from build123d import *

# Parameters (mm, degrees)
F0_W     = 406.4
F0_H     = 431.8
F1_DEPTH = 431.8
F2_W     = 304.8
F2_H     = 330.2
F3_DEPTH = 1270
F4_W     = 304.8
F4_H     = 330.2
F5_DEPTH = 754.38
F6_W     = 330.2
F6_H     = 330.2
F7_DEPTH = 1270


with BuildPart() as f1:
    # F0 (on Top) → F1 (new body)
    with BuildSketch(Plane.XY):
        with Locations((142.597137, -170.802241)):
            Rectangle(F0_W, F0_H)
    extrude(amount=F1_DEPTH)

    # F2 (on face) → F3 (cut)
    with BuildSketch(Plane.XZ.offset(386.702241)):
        with Locations((142.597137, 215.9)):
            Rectangle(F2_W, F2_H)
    extrude(amount=-F3_DEPTH, mode=Mode.SUBTRACT)

    # F4 (on face) → F5 (cut)
    with BuildSketch(Plane(origin=(0, 0, 0), x_dir=(1, 0, 0), z_dir=(0, 0, -1))):
        with Locations((142.597137, 170.802241)):
            Rectangle(F4_W, F4_H)
    extrude(amount=-F5_DEPTH, mode=Mode.SUBTRACT)

    # F6 (on face) → F7 (cut)
    with BuildSketch(Plane.YZ.offset(345.797137)):
        with Locations((-170.802241, 215.9)):
            Rectangle(F6_W, F6_H)
    extrude(amount=-F7_DEPTH, mode=Mode.SUBTRACT)


solid = f1.part
Input: part model. Units: mm. Frame: model coordinates. A direction names the side the tool comes from. Coordinates: 2 decimals unless noted, no trailing zeros. Loops run counter-clockwise (first coordinate to the right, second up) from the corner with the lowest first, then second, coordinate; pieces in that order, holes last.
Q1. Cut plane A-A (y = -231). Output: boundary loops of the cut face in (x, z), then the cut area to 3 significant figures.
Q2. Cut plane B-B (z = 347). Output: boundary loops of the cut face in (x, y), then the cut area to 3 significant figures.
Q3. Draft query along X for faces 1 (the face through (345.797, -366, 213)), 2 (the face through (321, -173, 50.8)), 3 (the face through (-9.803, 19, 214)). Return one class per face: +X half, -X half, draft (parallel to the pull), parting line (faces both ways), or undercut.
Q4. Material intervals for line 1 (X direction, y = -276, z = 27); line 2 (Z direction, x = 210.5, y = -339.5); line 3 (Y direction, x = 323, z = 317), sorted ascending.
Q5. Set-up query: faces 4 (the face through (294.997, 19, 214)), 5 (the face through (140, -5.702, 25)), 6 (the face through (321, -173, 381)). Return all of +Z, -Z, +X, -X, +Y, -Y with unobstructed straight access to the full face (end or side cutting, diameter ignored); none if empty.
Q6. Cut plane C-C (x = 301.5). Output: boundary loops of the cut face in (y, z).
Q7. Contact query for a flat-ended pin moving along its axis: pin 1 (6 mm diameter, centred on x = -6, z = 320, fed in from +Y). Output: stop coordinate, or through.
Working result:
1. outline: (-60.6, 0) - (-9.8, 0) - (-9.8, 50.8) - (-60.6, 50.8) - close; (-60.6, 381) - (-9.8, 381) - (-9.8, 431.8) - (-60.6, 431.8) - close; (295, 0) - (345.8, 0) - (345.8, 50.8) - (295, 50.8) - close; (295, 381) - (345.8, 381) - (345.8, 431.8) - (295, 431.8) - close
1. area: 10,300 mm2
2. outline: (-60.6, -386.7) - (-9.8, -386.7) - (-9.8, -335.9) - (-60.6, -335.9) - close; (-60.6, -5.7) - (-9.8, -5.7) - (-9.8, 45.1) - (-60.6, 45.1) - close; (295, -386.7) - (345.8, -386.7) - (345.8, -335.9) - (295, -335.9) - close; (295, -5.7) - (345.8, -5.7) - (345.8, 45.1) - (295, 45.1) - close
2. area: 10,300 mm2
3. face 1: +X half
3. face 2: draft
3. face 3: undercut
4. line 1: x = -60.6 to -9.8, 295 to 345.8
4. line 2: z = 0 to 50.8, 381 to 431.8
4. line 3: y = -386.7 to -335.9, -5.7 to 45.1
5. face 4: +Y, -Y
5. face 5: +Z, -Z
5. face 6: +X, -X
6. outline: (-386.7, 0) - (45.1, 0) - (45.1, 431.8) - (-386.7, 431.8) - close; hole (-335.9, 50.8) - (-5.7, 50.8) - (-5.7, 381) - (-335.9, 381) - close
7. pin 1: passes through
